Build history of the part. All positions in model axes, mm. A direction names the side the tool comes from. Coordinates: 2 decimals unless noted, no trailing zeros. Loops run counter-clockwise (first coordinate to the right, second up) from the corner with the lowest first, then second, coordinate; pieces in that order, holes last.
Item 1: Mould opens along X. For faces 1 (the face through (19.866, 37.164, 37.417)), 2 (the face through (15, 11, 39.389)), 3 (the face through (0.713, -2.809, -3.428)) say: released by +X, released by -X, zero draft, split by the parting line, or undercut.
Item 2: Flat gauge pins, fed straight in: pin 1 (6.5 mm diameter, centred on x = 4.56, y = 23.01, fed in from -Z); pin 2 (6.5 mm diameter, centred on x = 5.3, z = 26.52, fed in from -Y); pin 3 (6.5 mm diameter, centred on x = 34.5, z = 2.62, fed in from +Y); pin 4 (3 mm diameter, centred on x = 34, y = 2.5, fed in from -Z). Where does each tip first touch, or does it go through?
Item 3: Cut at A-A (x = 35.5). List the corners of the cut face in (y, z), and give its area (3 significant figures).
Item 4: Cut at D-D (x = 16). List the corners of the cut face in (y, z).
Item 5: Drill centre lines: line 1 along Y through (x, z) = (12.5, 36.4); line 2 along Y through (x, z) = (12, 37); line 3 along Z through (x, y) = (27, 14). Where is each one in solid material? Low to high.
Item 6: Cut at C-C (y = 27). List the corners of the cut face in (x, z), and give its area (3 significant figures).
Item 7: 3-axis set-ups, long thin cutter, end or side, ignore diameter. For faces 4 (the face through (29, 18, 35.389)), 5 (the face through (4, -3, 25)), 6 (the face through (26.1, 23, 37)): which of +Z, -Z, +X, -X, +Y, -Y reach the whole face in a straight line?
Item 8: Cut at B-B (z = 27). List the corners of the cut face in (x, y).
from build123d import *

# Parameters (mm, degrees)
SKETCH2_W           = 1.5
SKETCH2_H           = 37.57
SKETCH2_H_2         = 1.5
SKETCH2_W_2         = 39.569
BOSS_EXTRUDE1_DEPTH = 40
SKETCH3_R           = 1.65
CUT_EXTRUDE1_DEPTH  = 40
SKETCH4_R           = 10.5
SKETCH4_R_2         = 1.65
CUT_EXTRUDE2_DEPTH  = 40
SKETCH_1_R          = 10.5
SKETCH_1_R_2        = 1.65
EXTRUDE_1_DEPTH     = 2.5
FILLET_1_R          = 2.5
SKETCH_2_W          = 40
SKETCH_2_H          = 43.569
SKETCH_2_R          = 1.65
EXTRUDE_2_DEPTH     = 2
FILLET_2_R          = 2.5
SKETCH_3_R          = 1.65
EXTRUDE_3_DEPTH     = 3.5
SKETCH_4_R          = 2
CUT_EXTRUDE_1_DEPTH = 3.5
FILLET_3_R          = 3
SKETCH_5_W          = 40
SKETCH_5_H          = 4
EXTRUDE_4_DEPTH     = 27
FILLET_4_R          = 3
EXTRUDE_5_DEPTH     = 4
CUT_EXTRUDE_2_DEPTH = 4
SKETCH_10_R         = 2
CUT_EXTRUDE_3_DEPTH = 4


with BuildPart() as part:
    # Sketch2 → Boss-Extrude1 (new body)
    with BuildSketch(Plane(origin=(0, 0, 0), x_dir=(0, 0, -1), z_dir=(1, 0, 0))):
        with Locations((-36.139408466, 17.750517241)):
            Rectangle(SKETCH2_W, SKETCH2_H)
        with Locations((-36.139408466, -1.784482759)):
            Rectangle(SKETCH2_W, SKETCH2_H_2)
        with Locations((-15.604908466, -1.784482759)):
            Rectangle(SKETCH2_W_2, SKETCH2_H_2)
    extrude(amount=BOSS_EXTRUDE1_DEPTH)

    # Sketch3 → Cut-Extrude1 (cut)
    with BuildSketch(Plane(origin=(0, -1.034482759, 0), x_dir=(1, 0, 0), z_dir=(0, 1, 0))):
        with Locations(Location((4.5, -30.820408466, 0), (0, 0, 270))):
            Circle(SKETCH3_R)
        with Locations(Location((4.5, -20.820408466, 0), (0, 0, 270))):
            Circle(SKETCH3_R)
        with Locations(Location((4.5, -10.820408466, 0), (0, 0, 270))):
            Circle(SKETCH3_R)
        with Locations(Location((4.5, -0.820408466, 0), (0, 0, 270))):
            Circle(SKETCH3_R)
        with Locations(Location((35.5, -30.820408466, 0), (0, 0, 270))):
            Circle(SKETCH3_R)
        with Locations(Location((35.5, -20.820408466, 0), (0, 0, 270))):
            Circle(SKETCH3_R)
        with Locations(Location((35.5, -10.820408466, 0), (0, 0, 270))):
            Circle(SKETCH3_R)
        with Locations(Location((35.5, -0.820408466, 0), (0, 0, 270))):
            Circle(SKETCH3_R)
    extrude(amount=-CUT_EXTRUDE1_DEPTH, mode=Mode.SUBTRACT)

    # Sketch4 → Cut-Extrude2 (cut)
    with BuildSketch(Plane(origin=(0, 0, 35.389408466), x_dir=(-1, 0, 0), z_dir=(0, 0, -1))):
        with Locations(Location((-20, 16.535517241, 0), (0, 0, 90))):
            Circle(SKETCH4_R)
        with Locations(Location((-11.070998723, 25.983952889, 0), (0, 0, 90))):
            Circle(SKETCH4_R_2)
        with Locations(Location((-10.551564352, 7.606515964, 0), (0, 0, 90))):
            Circle(SKETCH4_R_2)
        with Locations(Location((-29.448435648, 25.464518519, 0), (0, 0, 90))):
            Circle(SKETCH4_R_2)
        with Locations(Location((-28.929001277, 7.087081594, 0), (0, 0, 90))):
            Circle(SKETCH4_R_2)
        with BuildLine():
            Line((-40, 36.535517241), (-40, 16.535517241))
            ThreePointArc((-40, 16.535517241), (-34.142135624, 30.677652865), (-20, 36.535517241))
            Line((-20, 36.535517241), (-40, 36.535517241))
        make_face()
        with BuildLine():
            Line((0, 36.535517241), (-20, 36.535517241))
            ThreePointArc((-20, 36.535517241), (-5.857864785, 30.677653274), (0, 16.535518399))
            Line((0, 16.535518399), (0, 36.535517241))
        make_face()
    extrude(amount=-CUT_EXTRUDE2_DEPTH, mode=Mode.SUBTRACT)

    # 草图1 → 凸台-拉伸1 (add)
    with BuildSketch(Plane.XY.offset(36.889408466)):
        with BuildLine():
            Line((0, 16.535517241), (0, -2.534482759))
            Line((0, -2.534482759), (40, -2.534482759))
            Line((40, -2.534482759), (40, 16.535517241))
            ThreePointArc((40, 16.535517241), (20, 36.535517241), (0, 16.535517241))
        make_face()
        with Locations(Location((20, 16.535517241, 0), (0, 0, 90))):
            Circle(SKETCH_1_R, mode=Mode.SUBTRACT)
        with Locations(Location((11.070998723, 25.983952889, 0), (0, 0, 90))):
            Circle(SKETCH_1_R_2, mode=Mode.SUBTRACT)
        with Locations(Location((29.448435648, 25.464518519, 0), (0, 0, 90))):
            Circle(SKETCH_1_R_2, mode=Mode.SUBTRACT)
        with Locations(Location((28.929001277, 7.087081594, 0), (0, 0, 90))):
            Circle(SKETCH_1_R_2, mode=Mode.SUBTRACT)
        with Locations(Location((10.551564352, 7.606515964, 0), (0, 0, 90))):
            Circle(SKETCH_1_R_2, mode=Mode.SUBTRACT)
    extrude(amount=EXTRUDE_1_DEPTH)

    # 圆角1
    fillet_1_edges = [part.edges().sort_by_distance(p)[0] for p in [
        (20, -1.034482759, 35.389408466),
    ]]
    fillet(fillet_1_edges, radius=FILLET_1_R)

    # 草图2 → 凸台-拉伸2 (add)
    with BuildSketch(Plane.XZ.offset(2.534482759)):
        with Locations((20, 17.604908466)):
            Rectangle(SKETCH_2_W, SKETCH_2_H)
        with Locations(Location((4.5, 30.820408466, 0), (0, 0, 90))):
            Circle(SKETCH_2_R, mode=Mode.SUBTRACT)
        with Locations(Location((4.5, 20.820408466, 0), (0, 0, 90))):
            Circle(SKETCH_2_R, mode=Mode.SUBTRACT)
        with Locations(Location((4.5, 0.820408466, 0), (0, 0, 90))):
            Circle(SKETCH_2_R, mode=Mode.SUBTRACT)
        with Locations(Location((4.5, 10.820408466, 0), (0, 0, 90))):
            Circle(SKETCH_2_R, mode=Mode.SUBTRACT)
        with Locations(Location((35.5, 30.820408466, 0), (0, 0, 90))):
            Circle(SKETCH_2_R, mode=Mode.SUBTRACT)
        with Locations(Location((35.5, 20.820408466, 0), (0, 0, 90))):
            Circle(SKETCH_2_R, mode=Mode.SUBTRACT)
        with Locations(Location((35.5, 10.820408466, 0), (0, 0, 90))):
            Circle(SKETCH_2_R, mode=Mode.SUBTRACT)
        with Locations(Location((35.5, 0.820408466, 0), (0, 0, 90))):
            Circle(SKETCH_2_R, mode=Mode.SUBTRACT)
    extrude(amount=EXTRUDE_2_DEPTH)

    # 圆角2
    fillet_2_edges = [part.edges().sort_by_distance(p)[0] for p in [
        (40, -3.534482759, -4.179591534),
        (0, -3.534482759, -4.179591534),
    ]]
    fillet(fillet_2_edges, radius=FILLET_2_R)

    # 草图3 → 凸台-拉伸3 (add)
    with BuildSketch(Plane(origin=(0, -1.034482759, 0), x_dir=(1, 0, 0), z_dir=(0, 1, 0))):
        with Locations((35.5, -0.820408466)):
            Circle(SKETCH_3_R)
        with Locations((35.5, -10.820408466)):
            Circle(SKETCH_3_R)
        with Locations((35.5, -20.820408466)):
            Circle(SKETCH_3_R)
        with Locations((35.5, -30.820408466)):
            Circle(SKETCH_3_R)
        with Locations((4.5, -0.820408466)):
            Circle(SKETCH_3_R)
        with Locations((4.5, -10.820408466)):
            Circle(SKETCH_3_R)
        with Locations((4.5, -20.820408466)):
            Circle(SKETCH_3_R)
        with Locations((4.5, -30.820408466)):
            Circle(SKETCH_3_R)
    extrude(amount=-EXTRUDE_3_DEPTH)

    # 草图4 → 切除-拉伸1 (cut)
    with BuildSketch(Plane(origin=(0, -1.034482759, 0), x_dir=(1, 0, 0), z_dir=(0, 1, 0))):
        with Locations(Location((34.5, -2.620408466, 0), (0, 0, 270))):
            Circle(SKETCH_4_R)
        with Locations(Location((34.5, -26.520408466, 0), (0, 0, 270))):
            Circle(SKETCH_4_R)
        with Locations(Location((5.3, -2.620408466, 0), (0, 0, 270))):
            Circle(SKETCH_4_R)
        with Locations(Location((5.3, -26.520408466, 0), (0, 0, 270))):
            Circle(SKETCH_4_R)
    extrude(amount=-CUT_EXTRUDE_1_DEPTH, mode=Mode.SUBTRACT)

    # 圆角3
    fillet_3_edges = [part.edges().sort_by_distance(p)[0] for p in [
        (20, -4.534482759, 39.389408466),
    ]]
    fillet(fillet_3_edges, radius=FILLET_3_R)

    # 草图5 → 凸台-拉伸4 (add)
    with BuildSketch(Plane.XZ.offset(4.534482759)):
        with Locations((20, 37.389408466)):
            Rectangle(SKETCH_5_W, SKETCH_5_H)
    extrude(amount=-EXTRUDE_4_DEPTH)

    # 圆角4
    fillet_4_edges = [part.edges().sort_by_distance(p)[0] for p in [
        (20, -4.534482759, 39.389408466),
    ]]
    fillet(fillet_4_edges, radius=FILLET_4_R)

    # 草图7 → 凸台-拉伸5 (add)
    with BuildSketch(Plane.XY.offset(39.389408466)):
        with BuildLine():
            Line((0, 22.465517241), (40, 22.465517241))
            ThreePointArc((40, 22.465517241), (20, 42.465517241), (0, 22.465517241))
        make_face()
    extrude(amount=-EXTRUDE_5_DEPTH)

    # 草图8 → 切除-拉伸2 (cut)
    with BuildSketch(Plane.XY.offset(39.389408466)):
        with BuildLine():
            Line((26.1, 31.065517241), (26.1, 15.465517241))
            ThreePointArc((26.1, 15.465517241), (20, 9.365517241), (13.9, 15.465517241))
            Line((13.9, 15.465517241), (13.9, 31.065517241))
            ThreePointArc((13.9, 31.065517241), (20, 37.165517241), (26.1, 31.065517241))
        make_face()
    extrude(amount=-CUT_EXTRUDE_2_DEPTH, mode=Mode.SUBTRACT)

    # 草图10 → 切除-拉伸3 (cut)
    with BuildSketch(Plane.XY.offset(39.389408466)):
        with Locations((12.5, 9.765517241)):
            Circle(SKETCH_10_R)
        with Locations((27.941342951, 10.020326713)):
            Circle(SKETCH_10_R)
        with Locations((35.441342951, 23.520326713)):
            Circle(SKETCH_10_R)
        with Locations((27.5, 36.765517241)):
            Circle(SKETCH_10_R)
        with Locations((12.058657049, 36.51070777)):
            Circle(SKETCH_10_R)
        with Locations((4.558657049, 23.01070777)):
            Circle(SKETCH_10_R)
    extrude(amount=-CUT_EXTRUDE_3_DEPTH, mode=Mode.SUBTRACT)


solid = part.part
Filled sheet:
1. face 1: undercut
1. face 2: zero draft
1. face 3: released by -X
2. pin 1: stops at z = 35.39
2. pin 2: stops at y = -4.53
2. pin 3: stops at y = -1.03
2. pin 4: stops at z = 35.35
3. outline: (-4.53, -4.18) - (-1.03, -4.18) - (-1.03, 0.89) - (-4.53, 0.89) - close; (-4.53, 4.35) - (-1.03, 4.35) - (-1.03, 24.79) - (-4.53, 24.79) - close; (-4.53, 28.25) - (-1.03, 28.25) - (-1.03, 32.89) arc R2.5 cw to (1.47, 35.39) - (21.52, 35.39) - (21.52, 39.39) - (-1.53, 39.39) arc R3 ccw to (-4.53, 36.39) - close; (25.52, 35.39) - (35.1, 35.39) - (35.1, 39.39) - (25.52, 39.39) - close
3. area: 256 mm2
4. outline: (-4.53, -4.18) - (-1.03, -4.18) - (-1.03, 32.89) arc R2.5 cw to (1.47, 35.39) - (10.86, 35.39) - (10.86, 39.39) - (-1.53, 39.39) arc R3 ccw to (-4.53, 36.39) - close; (35.67, 35.39) - (42.06, 35.39) - (42.06, 39.39) - (35.67, 39.39) - close
5. line 1: y = -4.53 to 7.77, 11.77 to 34.56, 38.46 to 41.01
5. line 2: y = -4.47 to 7.83, 11.7 to 34.51, 38.51 to 40.8
5. line 3: z = 35.39 to 39.39
6. outline: (0.52, 35.39) - (13.9, 35.39) - (13.9, 39.39) - (0.52, 39.39) - close; (26.1, 35.39) - (39.48, 35.39) - (39.48, 39.39) - (26.1, 39.39) - close
6. area: 107 mm2
7. face 4: -Z, +X, -X, +Y
7. face 5: +Y, -Y
7. face 6: +Z, -Z
8. outline: (0, -4.53) - (3.36, -4.53) - (3.36, -1.03) - (0, -1.03) - close; (7.24, -4.53) - (32.56, -4.53) - (32.56, -1.03) - (7.24, -1.03) - close; (36.44, -4.53) - (40, -4.53) - (40, -1.03) - (36.44, -1.03) - close
